from build123d import *

# Parameters (mm, degrees)
F1_DEPTH  = 10
F3_DEPTH  = 10.001
F4_R      = 5.5
F4_R_2    = 4.25
F5_DEPTH  = 2
F6_DEPTH  = 112.584302492
F7_R      = 1.395
F8_DEPTH  = 1.5
F9_DEPTH  = 25
F11_DEPTH = 3


with BuildPart() as f1:
    # F0 (on Front) → F1 (new body, symmetric)
    with BuildSketch(Plane.XZ):
        with BuildLine():
            Line((30, 51.9615242271), (0, 0))
            Line((0, 0), (130, 0))
            Line((130, 0), (130, 10))
            Line((130, 10), (88.0384757729, 10))
            ThreePointArc((88.0384757729, 10), (82.8620948709, 10.6814834742), (78.0384757729, 12.6794919243))
            Line((78.0384757729, 12.6794919243), (62.2390923627, 21.8012701892))
            ThreePointArc((62.2390923627, 21.8012701892), (61.5402036233, 22.7120797272), (61.6900542571, 23.8503082949))
            Line((61.6900542571, 23.8503082949), (44.3695461814, 33.8503082949))
            ThreePointArc((44.3695461814, 33.8503082949), (43.4587366433, 33.1514195555), (42.3205080757, 33.3012701892))
            Line((42.3205080757, 33.3012701892), (27.5980762114, 41.8012701892))
            ThreePointArc((27.5980762114, 41.8012701892), (26.8991874719, 42.7120797272), (27.0490381057, 43.8503082949))
            Line((27.0490381057, 43.8503082949), (31.2990381057, 51.2115242271))
            Line((31.2990381057, 51.2115242271), (30, 51.9615242271))
        make_face()
        with BuildLine():
            Line((11.2990381057, 16.5705080757), (23.0490381057, 36.9221050646))
            ThreePointArc((23.0490381057, 36.9221050646), (26.0850698991, 39.2517341961), (29.8791651246, 38.7522320835))
            Line((29.8791651246, 38.7522320835), (78.2416697508, 10.8301270189))
            ThreePointArc((78.2416697508, 10.8301270189), (80.5712988822, 5.2059047745), (75.7416697508, 1.5))
            Line((75.7416697508, 1.5), (27.4019237886, 1.5))
            Line((27.4019237886, 1.5), (13.1291651246, 9.7403810568))
            ThreePointArc((13.1291651246, 9.7403810568), (10.7995359932, 12.7764128502), (11.2990381057, 16.5705080757))
        make_face(mode=Mode.SUBTRACT)
    extrude(amount=F1_DEPTH, both=True)

    # F2 (on face) → F3 (cut, through all)
    with BuildSketch(Plane.XY.offset(10)):
        with BuildLine():
            Line((130, -10), (130, -5))
            Line((130, -5), (98, -5))
            ThreePointArc((98, -5), (95.8786796564, -5.8786796564), (95, -8))
            Line((95, -8), (95, -10))
            Line((95, -10), (130, -10))
        make_face()
        with BuildLine():
            Line((130, -3), (130, 3))
            Line((130, 3), (113, 3))
            ThreePointArc((113, 3), (110, 0), (113, -3))
            Line((113, -3), (130, -3))
        make_face()
        with BuildLine():
            Line((98, 5), (130, 5))
            Line((130, 5), (130, 10))
            Line((130, 10), (95, 10))
            Line((95, 10), (95, 8))
            ThreePointArc((95, 8), (95.8786796564, 5.8786796564), (98, 5))
        make_face()
    extrude(amount=-F3_DEPTH, mode=Mode.SUBTRACT)

    # F4 (on face) → F5 (cut)
    with BuildSketch(Plane(origin=(0, 0, 0), x_dir=(0, -1, 0), z_dir=(-0.8660254038, 0, 0.5))):
        with Locations((0, 7.5)):
            Circle(F4_R)
        with Locations((0, 7.5)):
            Circle(F4_R_2, mode=Mode.SUBTRACT)
    extrude(amount=-F5_DEPTH, mode=Mode.SUBTRACT)

    # F6 (cut, through all): a face of the model
    f6_faces = [f1.faces().sort_by_distance(p)[0] for p in [
        (3.75, 0, 6.4951905284),
    ]]
    extrude(f6_faces, amount=-F6_DEPTH, mode=Mode.SUBTRACT)

    # F7 (on face) → F8 (cut, through all)
    with BuildSketch(Plane(origin=(0, 0, 0), x_dir=(0, -1, 0), z_dir=(-0.8660254038, 0, 0.5))):
        with Locations((-5, 32)):
            Circle(F7_R)
        with Locations((-5, 25)):
            Circle(F7_R)
        with Locations((-5, 39)):
            Circle(F7_R)
    extrude(amount=-F8_DEPTH, mode=Mode.SUBTRACT)

    # F7 (on face) → F9 (cut)
    with BuildSketch(Plane(origin=(0, 0, 0), x_dir=(0, -1, 0), z_dir=(-0.8660254038, 0, 0.5))):
        with Locations((-5, 25)):
            Circle(F7_R)
        with Locations((-5, 32)):
            Circle(F7_R)
        with Locations((-5, 39)):
            Circle(F7_R)
        with Locations((5, 39)):
            Circle(F7_R)
        with Locations((5, 32)):
            Circle(F7_R)
        with Locations((5, 25)):
            Circle(F7_R)
    extrude(amount=-F9_DEPTH, mode=Mode.SUBTRACT)

    # F10 (on face) → F11 (cut, through all)
    with BuildSketch(Plane(origin=(25.75, 0, 44.6003082949), x_dir=(0.8660254038, 0, -0.5), z_dir=(0.5, 0, 0.8660254038))):
        with BuildLine():
            ThreePointArc((27.9322247952, 4), (23.9322247952, 0), (27.9322247952, -4))
            Line((27.9322247952, -4), (34.9322247952, -4))
            ThreePointArc((34.9322247952, -4), (38.9322247952, 0), (34.9322247952, 4))
            Line((34.9322247952, 4), (27.9322247952, 4))
        make_face()
    extrude(amount=-F11_DEPTH, mode=Mode.SUBTRACT)


solid = f1.part
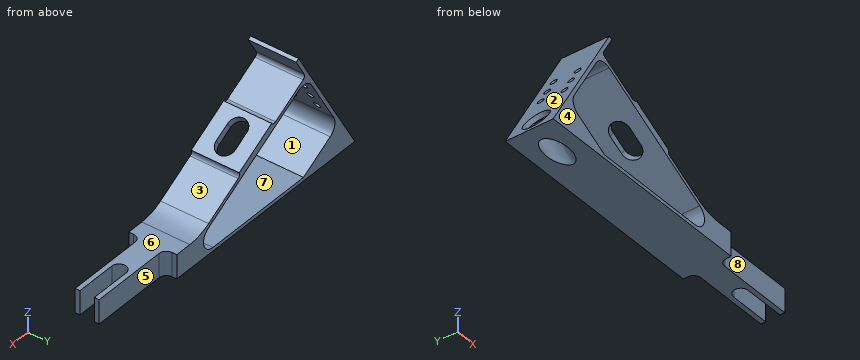
Geometry check sheet. Reference: the model listing, model coordinates, mm. Face numbers are marked on the shaded views. A direction names the side the tool comes from. Coordinates: 2 decimals unless noted, no trailing zeros. Order: outer loops, then holes, each group sorted by start corner. A loop starts at its lowest first (then second) coordinate and runs counter-clockwise, first axis right, second up. Notation, with made-up numbers: (-9, 14.25) -> (38, 14.25) arc R19 cw to (38, 33.25) -> close; hole circle Ø9 at (-33.5, 58.5). An arc over 180 degrees is marked (long way). Use a Markdown table: item, result. Add a question column.
1. Cross-section at A-A (x = 119). Enter the section's corners in (y, z).
2. Cross-section at C-C (x = 68.5). Enter the section's corners in (y, z), and give its area (3 significant figures).
3. Go/stop test with flat-tipped pins: pin 1 Ø8 at (y, z) = (7.5, 21.5) entering from +X; pin 2 Ø3 at (x, z) = (120.5, 2.5) entering from +Y; pin 3 Ø5 at (y, z) = (-5.5, 44) entering from -X. Record where each tip stops, or that it passes through.
4. Cross-section at D-D (z = 48.5). Enter the section's corners in (x, y), and give its area (3 significant figures).
5. Cross-section at B-B (x = 104.5). Enter the section's corners in (y, z).
6. Mould release check, pull along X, two halves, no side actions. Record for the marked faces 1, 2, 3 and 4: pulls with the +X half, pulls with the -X half, needs draft (parallel to the pull), parting line crosses it, or undercut.
7. Set-up check for the marked faces 5, 6, 7 and 8: record each of +Z, -Z, +X, -X, +Y, -Y from which the full face is reachable in a straight line by a thin tool's end or side.
8. Material ranges on L1, parallel to Y at x = 102, z = 6.5; L2, parallel to Z at x = 50.5, y = -2.25; L3, parallel to Z at x = 19, y = 9.25, recorded low to high.
Filled sheet:
| question | item | result |
|---|---|---|
| 1 | outline | (-5, 0) -> (-3, 0) -> (-3, 10) -> (-5, 10) -> close; (3, 0) -> (5, 0) -> (5, 10) -> (3, 10) -> close |
| 2 | outline | (-10, 0) -> (10, 0) -> (10, 1.5) -> (-10, 1.5) -> close; (-10, 16.45) -> (10, 16.45) -> (10, 18.19) -> (-10, 18.19) -> close |
| 2 | area | 64.6 mm2 |
| 3 | pin 1 | x = 69.69 |
| 3 | pin 2 | y = 5 |
| 3 | pin 3 | x = 23.96 |
| 4 | outline | (28, -10) -> (29.73, -10) -> (29.73, 10) -> (28, 10) -> close |
| 4 | area | 34.6 mm2 |
| 5 | outline | (-5, 0) -> (5, 0) -> (5, 10) -> (-5, 10) -> close |
| 6 | face 1 | undercut |
| 6 | face 2 | pulls with the -X half |
| 6 | face 3 | pulls with the +X half |
| 6 | face 4 | needs draft |
| 7 | face 5 | +Z, -Z, +X, +Y |
| 7 | face 6 | +Z, +X, +Y, -Y |
| 7 | face 7 | +Y, -Y |
| 7 | face 8 | +Z, -Z, +X, -Y |
| 8 | L1 | -5 to 5 |
| 8 | L2 | 0 to 1.5 |
| 8 | L3 | 0 to 6.35, 29.91 to 32.91 |
